Design review of the part built by this model. Coordinates are the model's own, in mm. A direction names the side the tool comes from. Coordinates: 2 decimals unless noted, no trailing zeros. Write each loop counter-clockwise with the first axis right and the second up, starting at its lowest first coordinate (ties: lowest second). Pieces come first, ordered by that corner, then holes.
Q1. Add section B-B, the plane x = -1. Give the boundary of the cut face in (y, z).
Q2. The part is to be moulded in two halves that separate along Z. For faces 1 (the face through (1, 5, 10)), 2 (the face through (-4, 13, 5)), 3 (the face through (2.535, -20.555, 21.741)), say which applies: +Z half, -Z half, draft (parallel to the pull), parting line (faces both ways), or undercut.
Q3. Add section A-A, the plane y = 7.5. Give the boundary of the cut face in (x, z), plus the area to 3 significant figures.
Q4. Machinability: for faces 4 (the face through (-0.54, -39.94, 4.93)), 5 (the face through (-4, -28, 23)), 6 (the face through (-4, -2, 23)), 7 (the face through (3, -1, 23)), 8 (the face through (3, -29, 23)), which of the approach directions +Z, -Z, +X, -X, +Y, -Y give a long, thin tool a straight path to every point of the face, cutting with its end or side? Answer none if there is none.
Q5. Clearance check with flat-ended pins moving along their axes: pin 1 Ø12.5 at (y, z) = (-15, 26) entering from +X; pin 2 Ø5 at (x, y) = (1, 8.5) entering from +Z; pin 3 Ø1.5 at (x, z) = (0.5, 20.5) entering from +Y. State where each tip first meets the part, or that it passes through.
Q6. To check wall thickness, follow probe 1 along Y at (x, z) = (0, 5.25); probe 2 along X at (y, z) = (-17.5, 19.5); probe 3 along Z at (x, y) = (-3.5, -17.5). State the ranges of each line that lie inside material, in increasing order.
from build123d import *

# Parameters (mm, degrees)
F0_W     = 10
F0_H     = 30
F1_DEPTH = 40
F0_H_2   = 15
F0_R     = 2.5
F2_DEPTH = 10
F3_R     = 5
F4_DEPTH = 25
F3_R_2   = 7
F5_DEPTH = 5
F6_R     = 4.99999
F7_R     = 4.99999


# Not quite as in the source:
# - a fillet or chamfer is up to 0.001 mm smaller than in the source, because OpenCascade refuses the exact size


with BuildPart() as f1:
    # F0 (on Top) → F1 (new body)
    with BuildSketch(Plane.XY):
        with Locations((0, -15)):
            Rectangle(F0_W, F0_H)
    extrude(amount=F1_DEPTH)

    # F0 (on Top) → F2 (join)
    with BuildSketch(Plane.XY):
        with Locations((0, 7.5)):
            Rectangle(F0_W, F0_H_2)
        with Locations((0, 7.5)):
            Circle(F0_R, mode=Mode.SUBTRACT)
        with Locations((0, -37.5)):
            Rectangle(F0_W, F0_H_2)
        with Locations((0, -37.5)):
            Circle(F0_R, mode=Mode.SUBTRACT)
    extrude(amount=F2_DEPTH)

    # F3 (on face) → F4 (cut)
    with BuildSketch(Plane.YZ.offset(5)):
        with Locations((-15, 26)):
            Circle(F3_R)
    extrude(amount=-F4_DEPTH, mode=Mode.SUBTRACT)

    # F3 (on face) → F5 (cut)
    with BuildSketch(Plane.YZ.offset(5)):
        with Locations((-15, 26)):
            Circle(F3_R_2)
        with Locations((-15, 26)):
            Circle(F3_R, mode=Mode.SUBTRACT)
    extrude(amount=-F5_DEPTH, mode=Mode.SUBTRACT)

    # F6 (radius 5 in the source; OpenCascade refuses exactly that, so slightly less here)
    f6_edges = [f1.edges().sort_by_distance(p)[0] for p in [
        (0, -30, 40),
        (5, -15, 40),
        (0, 0, 40),
        (-5, -15, 40),
        (5, 0, 25),
        (5, -30, 25),
        (-5, -30, 25),
        (-5, 0, 25),
    ]]
    fillet(f6_edges, radius=F6_R)

    # F7 (radius 5 in the source; OpenCascade refuses exactly that, so slightly less here)
    f7_edges = [f1.edges().sort_by_distance(p)[0] for p in [
        (5, 15, 5),
        (-5, 15, 5),
        (5, -45, 5),
        (-5, -45, 5),
    ]]
    fillet(f7_edges, radius=F7_R)


solid = f1.part
Here are the results:
1. outline: (-44.9, 0) - (-39.79, 0) - (-39.79, 10) - (-44.9, 10) - close; (-35.21, 0) - (5.21, 0) - (5.21, 10) - (-0.1, 10) - (-0.1, 35) arc R4.9 ccw to (-5, 39.9) - (-25, 39.9) arc R4.9 ccw to (-29.9, 35) - (-29.9, 10) - (-35.21, 10) - close; (9.79, 0) - (14.9, 0) - (14.9, 10) - (9.79, 10) - close; hole circle Ø10 at (-15, 26)
2. face 1: +Z half
2. face 2: draft
2. face 3: undercut
3. outline: (-5, 0) - (-2.5, 0) - (-2.5, 10) - (-5, 10) - close; (2.5, 0) - (5, 0) - (5, 10) - (2.5, 10) - close
3. area: 50.0 mm2
4. face 4: +Z, -Z
4. face 5: +Z, -X, -Y
4. face 6: +Z, -X, +Y
4. face 7: +Z, +X, +Y
4. face 8: +Z, +X, -Y
5. pin 1: stops at x = 0
5. pin 2: stops at z = 10
5. pin 3: stops at y = 0
6. probe 1: y = -45 to -40, -35 to 5, 10 to 15
6. probe 2: x = -5 to 0
6. probe 3: z = 0 to 21.67, 30.33 to 38.57
